from build123d import *

# Parameters (mm, degrees)
BOSS_EXTRUDE2_DEPTH = 1600
SKETCH3_R           = 40.5
CUT_EXTRUDE2_DEPTH  = 52


with BuildPart() as part:
    # Sketch2 → Boss-Extrude2 (new body)
    with BuildSketch(Plane(origin=(0, 0, 0), x_dir=(1, 0, 0), z_dir=(0, 1, 0))):
        Polygon((-22.5, 47.5), (25.5, 47.5), (25.5, 50.5), (-25.5, 50.5), (-25.5, -50.5), (25.5, -50.5), (25.5, -47.5), (-22.5, -47.5), align=None)
    extrude(amount=BOSS_EXTRUDE2_DEPTH)

    # Sketch3 → Cut-Extrude2 (cut, through all)
    with BuildSketch(Plane.ZY.offset(25.5)):
        with Locations((0, 50)):
            Circle(SKETCH3_R)
        with Locations((0, 1550)):
            Circle(SKETCH3_R)
    extrude(amount=-CUT_EXTRUDE2_DEPTH, mode=Mode.SUBTRACT)


solid = part.part
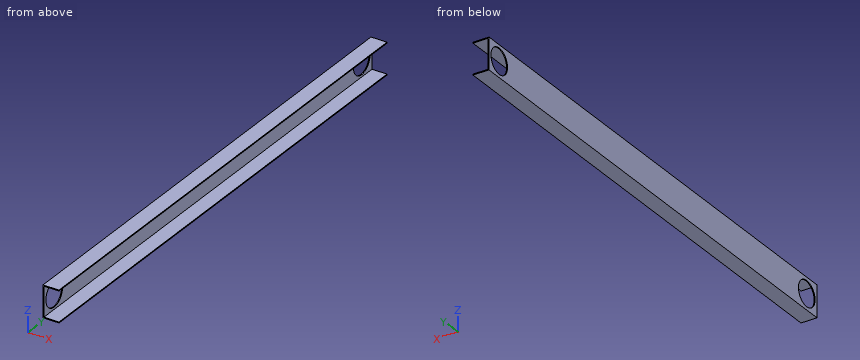
Geometry: final body of the model. Coordinates: model frame, mm. Round coordinates to 2 decimals unless told otherwise and drop trailing zeros. Order: outer loops, then holes, each group sorted by start corner. A loop starts at its lowest first (then second) coordinate and runs counter-clockwise, first axis right, second up. Notation, with made-up numbers: (40, -40) - (59, -40) arc R28 cw to (59, -4) - close; hole circle Ø9 at (20, -10). An arc over 180 degrees is marked (long way). Write each question's results on one line, items separated by ' | '.
Item 1: Material intervals for line 1 along Y through (x, z) = (-23, 0); line 2 along Z through (x, y) = (19, 393); line 3 along Y through (x, z) = (-23, -19.5), sorted ascending. Write a range as [from, to].
Completed:
line 1: [0, 9.5], [90.5, 1509.5], [1590.5, 1600] | line 2: [-50.5, -47.5], [47.5, 50.5] | line 3: [0, 14.5], [85.5, 1514.5], [1585.5, 1600]
Item 2: Section D-D, the plane y = 466. Return the cut outline in (x, z).
Completed:
outline: (-25.5, -50.5) - (25.5, -50.5) - (25.5, -47.5) - (-22.5, -47.5) - (-22.5, 47.5) - (25.5, 47.5) - (25.5, 50.5) - (-25.5, 50.5) - close
Item 3: Section C-C, the plane z = 0. Return the cut outline in (x, y), and give its area (3 significant figures).
Completed:
outline: (-25.5, 0) - (-22.5, 0) - (-22.5, 9.5) - (-25.5, 9.5) - close; (-25.5, 90.5) - (-22.5, 90.5) - (-22.5, 1509.5) - (-25.5, 1509.5) - close; (-25.5, 1590.5) - (-22.5, 1590.5) - (-22.5, 1600) - (-25.5, 1600) - close | area: 4,310 mm^2
Item 4: Section A-A, the plane y = 50. Return the cut outline in (x, z), and give its area (3 significant figures).
Completed:
outline: (-25.5, -50.5) - (25.5, -50.5) - (25.5, -47.5) - (-22.5, -47.5) - (-22.5, -40.5) - (-25.5, -40.5) - close; (-25.5, 40.5) - (-22.5, 40.5) - (-22.5, 47.5) - (25.5, 47.5) - (25.5, 50.5) - (-25.5, 50.5) - close | area: 348 mm^2
Item 5: Section B-B, the plane x = -8. Return the cut outline in (y, z).
Completed:
outline: (0, -50.5) - (1600, -50.5) - (1600, -47.5) - (0, -47.5) - close; (0, 47.5) - (1600, 47.5) - (1600, 50.5) - (0, 50.5) - close
Item 6: First-contact query: pin 1 Ø10 at (y, z) = (1343.5, -13.5) entering from +X. Flat tip, straight axial feed; report the tip coordinate or a pass-through.
Completed:
pin 1: x = -22.5
